The listing builds one solid part. Answer for the finished solid, in the listing's coordinates (mm). A direction names the side the tool comes from. Coordinates: 2 decimals unless noted, no trailing zeros. Write each loop counter-clockwise with the first axis right and the second up, starting at its lowest first coordinate (ties: lowest second). Pieces come first, ordered by that corner, then holes.
from build123d import *

# Parameters (mm, degrees)
F0_R      = 6.35
F1_DEPTH  = 11.049
F3_DEPTH  = 22.098
F5_DEPTH  = 12.7
F6_DEPTH  = 22.098
F8_DEPTH  = 12.7
F10_DEPTH = 228.6
F11_W     = 3.175
F11_H     = 50.8
F12_DEPTH = 31.75
F13_R     = 6.35
F14_DEPTH = 42.8


with BuildPart() as f1:
    # F0 (on Right) → F1 (new body, symmetric)
    with BuildSketch(Plane.YZ):
        with BuildLine():
            Line((1369.9610694916, 12.7), (-27.0389305084, 12.7))
            ThreePointArc((-27.0389305084, 12.7), (-39.7389305084, 0), (-27.0389305084, -12.7))
            Line((-27.0389305084, -12.7), (1369.9610694916, -12.7))
            ThreePointArc((1369.9610694916, -12.7), (1382.6610694916, 0), (1369.9610694916, 12.7))
        make_face()
        with Locations((-27.0389305084, 0)):
            Circle(F0_R, mode=Mode.SUBTRACT)
        with Locations((1369.9610694916, 0)):
            Circle(F0_R, mode=Mode.SUBTRACT)
    extrude(amount=F1_DEPTH, both=True)

    # F2 (on face) → F3 (join, through all)
    with BuildSketch(Plane.YZ.offset(11.049)):
        Polygon((1332.1480751038, -12.7), (8.231587708, -12.7), (271.9207406044, -66.1958232522), align=None)
    extrude(amount=-F3_DEPTH)

    # F4 (on face) → F5 (join)
    with BuildSketch(Plane.YZ.offset(11.049)):
        Polygon((1332.1480751038, 12.7), (8.231587708, 12.7), (8.231587708, -12.7), (271.9207406044, -66.1958232522), (1332.1480751038, -12.7), align=None)
        Polygon((271.9207406044, 26.0049468334), (8.231587708, 12.7), (1332.1480751038, 12.7), align=None)
    extrude(amount=F5_DEPTH)

    # F6 (add, through all): a face of the model
    f6_faces = [f1.faces().sort_by_distance(p)[0] for p in [
        (11.049, 537.4334678054, 17.1349822778),
    ]]
    extrude(f6_faces, amount=F6_DEPTH)

    # F7 (on face) → F8 (join)
    with BuildSketch(Plane(origin=(-11.049, 0, 0), x_dir=(0, -1, 0), z_dir=(-1, 0, 0))):
        Polygon((-1332.1480751038, 12.7), (-1332.1480751038, -12.7), (-271.9207406044, -66.1958232522), (-8.231587708, -12.7), (-8.231587708, 12.7), (-271.9207406044, 26.0049468334), align=None)
    extrude(amount=F8_DEPTH)

    # F9 (on Top) → F10 (cut, symmetric)
    with BuildSketch(Plane.XY):
        Polygon((-23.749, 570.2539157877), (-11.049, 1332.1480751038), (-42.6509715617, 1362.8944158554), (-507.5538158417, 214.9578332901), (-61.7056079209, -33.5918478668), (-11.049, 8.231587708), (-23.749, 163.8539157877), align=None)
        Polygon((23.749, 163.8539157877), (11.049, 8.231587708), (61.7056079209, -33.5918478668), (507.5538158417, 214.9578332901), (42.6509715617, 1362.8944158554), (11.049, 1332.1480751038), (23.749, 570.2539157877), align=None)
    extrude(amount=F10_DEPTH, both=True, mode=Mode.SUBTRACT)

    # F11 (on face) → F12 (join)
    with BuildSketch(Plane(origin=(0, 0.3691040914, 29.4126877667), x_dir=(1, 0, 0), z_dir=(0, 0.0125481573, 0.9999212688))):
        with Locations((-17.4625, 698.334315244)):
            Rectangle(F11_W, F11_H)
        with Locations((17.4625, 698.334315244)):
            Rectangle(F11_W, F11_H)
    extrude(amount=F12_DEPTH)

    # F13 (on face) → F14 (cut, through all)
    with BuildSketch(Plane.YZ.offset(19.05)):
        with BuildLine():
            Line((673.6488423855, 52.7161024408), (673.2504383927, 20.9686021572))
            Line((673.2504383927, 20.9686021572), (683.2025858499, 42.5725283176))
            ThreePointArc((683.2025858499, 42.5725283176), (689.7252525102, 49.7418257688), (699.0468426124, 52.3973792465))
            Line((699.0468426124, 52.3973792465), (673.6488423855, 52.7161024408))
        make_face()
        with Locations((699.0468426124, 34.7091633821)):
            Circle(F13_R)
        with BuildLine():
            Line((714.891099375, 42.5725283176), (724.0753566856, 22.6355229997))
            Line((724.0753566856, 22.6355229997), (724.4448428393, 52.0786560523))
            Line((724.4448428393, 52.0786560523), (699.4907166914, 52.3918090062))
            ThreePointArc((699.4907166914, 52.3918090062), (708.556331026, 49.6236734504), (714.891099375, 42.5725283176))
        make_face()
    extrude(amount=-F14_DEPTH, mode=Mode.SUBTRACT)


solid = f1.part
1. Section A-A on y = 373.5 is taken. Give the vertices of the cut face in (x, z), then the cut area to 3 significant figures.
Results found:
outline: (-23.75, -61.07) - (23.75, -61.07) - (23.75, 24.73) - (-23.75, 24.73) - close
area: 4,080 mm2
2. Section B-B on y = 917.5 is taken. Give the vertices of the cut face in (x, z).
Results found:
outline: (-17.96, -33.62) - (17.96, -33.62) - (17.96, 17.9) - (-17.96, 17.9) - close
3. Find the intervals of material crossed by L1, parallel to Z at x = 5.5, y = 570.5; L2, parallel to Z at x = 19, y = 156; L3, parallel to Y at x = 18, z = 31, in increasing order.
Results found:
L1: z = -51.13 to 22.26
L2: z = -42.68 to 20.16
L3: y = 677.87 to 693.89, 704.2 to 720.22
4. Flat-ended cylindrical pins translate along their axes: P1, Ø3, axis at y = 1120, z = -23, coming from the +X side; P2, Ø16, axis at y = 707.5, z = 35, coming from the +X side; P3, Ø20.5, axis at y = 699.05, z = 34.71, coming from the -X side. Find the tip coordinate at first contact, or state that the pin passes through.
Results found:
P1: stops at x = 14.61
P2: stops at x = 19.05
P3: stops at x = -19.05
5. A tool of negligible diameter and unlimited length cuts with its end or side. For faces 4 (the flat face through (-11.049, -11, 0)), 5 (the flat face through (19.05, 692.8, 32.8)), 6 (the flat face through (0, 1351, 12.7)), 7 (the flat face through (11.049, 1357, 0)), from which of +Z, -Z, +X, -X, +Y, -Y can it reach the whole face along a straight path? Write none if from no direction.
Results found:
face 4: +Z, -Z, -X, -Y
face 5: +Z, +X, +Y
face 6: +Z, +X, -X, +Y
face 7: +Z, -Z, +X, +Y
6. For a pull along X with two mould halves and no side action, classify faces 1 (the flat face through (-11.049, 1357, 0)), 2 (the flat face through (-15.875, 692.8, 32.8)), 3 (the flat face through (11.049, -11, 0)) as pulls with the +X half, pulls with the -X half, needs draft (parallel to the pull), parting line crosses it, or undercut.
Results found:
face 1: pulls with the -X half
face 2: undercut
face 3: pulls with the +X half
